Autodesk Inventor part; units mm, degrees
ref_plane "Work Plane2" through (2.8575, 0, 0) normal (1, 0, 0) x (0, 0, -1)
ref_plane "YZ Plane" through (0, 0, 0) normal (1, 0, 0) x (0, 1, 0)
ref_plane "XZ Plane" through (0, 0, 0) normal (0, 1, 0) x (-1, 0, 0)
ref_plane "Work Plane2" through (2.8575, 0, 0) normal (1, 0, 0) x (0, 0, -1)
sketch "Sketch6" plane through (2.8575, 0, 0) normal (1, 0, 0) x (0, 0, -1)
  line L0 (0.7654, -5.6784) -> (0.7654, -5.022)
  line L1 (-0.7638, -5.6784) -> (-0.7638, -5.0222)
  arc A0 (5.6006, 2.3498) -> (5.5837, 2.3418) centre (6.3532, 0.7382) ccw
  arc A1 (-0.7638, -5.0222) -> (0.7654, -5.022) centre (0, 0) ccw
  line L2 (0.0008, -7.62) -> (-0.2439, -7.62)
  line L3 (0.0008, -7.62) -> (0.2479, -7.62)
  arc A2 (0.2479, -7.62) -> (0.7654, -5.6784) centre (-2.309, -5.8988) ccw
  arc A3 (-0.7638, -5.6784) -> (-0.2439, -7.62) centre (2.2185, -5.9201) ccw
  arc A4 (3.5877, -3.5965) -> (3.5976, -3.5866) centre (0, 0) ccw
  line L4 (3.502, -4.5349) -> (3.1738, -3.9665)
  line L5 (2.1777, -5.2996) -> (1.8496, -4.7313)
  arc A5 (1.8496, -4.7313) -> (3.1738, -3.9665) centre (0, 0) ccw
  line L6 (3.8107, -6.5987) -> (3.5988, -6.721)
  line L7 (3.8107, -6.5987) -> (4.0247, -6.4752)
  arc A6 (4.0247, -6.4752) -> (3.502, -4.5349) centre (0.9498, -6.263) ccw
  arc A7 (2.1777, -5.2996) -> (3.5988, -6.721) centre (4.8813, -4.0177) ccw
  line L8 (5.3003, -2.1764) -> (4.7319, -1.8482)
  line L9 (4.5358, -3.5007) -> (3.9675, -3.1726)
  arc A8 (3.9675, -3.1726) -> (4.7319, -1.8482) centre (0, 0) ccw
  line L10 (6.5995, -3.8093) -> (6.4772, -4.0212)
  line L11 (6.5995, -3.8093) -> (6.7231, -3.5953)
  arc A9 (6.7231, -3.5953) -> (5.3003, -2.1764) centre (3.954, -4.949) ccw
  arc A10 (4.5358, -3.5007) -> (6.4772, -4.0212) centre (6.2362, -1.0388) ccw
  line L12 (5.6784, 0.7654) -> (5.022, 0.7654)
  line L13 (5.6784, -0.7638) -> (5.0222, -0.7638)
  arc A11 (5.0222, -0.7638) -> (5.022, 0.7654) centre (0, 0) ccw
  line L14 (7.62, 0.0008) -> (7.62, -0.2439)
  line L15 (7.62, 0.0008) -> (7.62, 0.2479)
  arc A12 (7.62, 0.2479) -> (5.6784, 0.7654) centre (5.8988, -2.309) ccw
  arc A13 (5.6784, -0.7638) -> (7.62, -0.2439) centre (5.9201, 2.2185) ccw
  line L16 (4.5349, 3.502) -> (3.9665, 3.1738)
  line L17 (5.2996, 2.1777) -> (4.7313, 1.8496)
  arc A14 (4.7313, 1.8496) -> (3.9665, 3.1738) centre (0, 0) ccw
  line L18 (6.5987, 3.8107) -> (6.721, 3.5988)
  line L19 (6.5987, 3.8107) -> (6.4752, 4.0247)
  arc A15 (6.4752, 4.0247) -> (4.5349, 3.502) centre (6.263, 0.9498) ccw
  arc A16 (5.2996, 2.1777) -> (6.721, 3.5988) centre (4.0177, 4.8813) ccw
  line L20 (2.1764, 5.3003) -> (1.8482, 4.7319)
  line L21 (3.5007, 4.5358) -> (3.1726, 3.9675)
  arc A17 (3.1726, 3.9675) -> (1.8482, 4.7319) centre (0, 0) ccw
  line L22 (3.8093, 6.5995) -> (4.0212, 6.4772)
  line L23 (3.8093, 6.5995) -> (3.5953, 6.7231)
  arc A18 (3.5953, 6.7231) -> (2.1764, 5.3003) centre (4.949, 3.954) ccw
  arc A19 (3.5007, 4.5358) -> (4.0212, 6.4772) centre (1.0388, 6.2362) ccw
  line L24 (-0.7654, 5.6784) -> (-0.7654, 5.022)
  line L25 (0.7638, 5.6784) -> (0.7638, 5.0222)
  arc A20 (0.7638, 5.0222) -> (-0.7654, 5.022) centre (0, 0) ccw
  line L26 (-0.0008, 7.62) -> (0.2439, 7.62)
  line L27 (-0.0008, 7.62) -> (-0.2479, 7.62)
  arc A21 (-0.2479, 7.62) -> (-0.7654, 5.6784) centre (2.309, 5.8988) ccw
  arc A22 (0.7638, 5.6784) -> (0.2439, 7.62) centre (-2.2185, 5.9201) ccw
  line L28 (-3.502, 4.5349) -> (-3.1738, 3.9665)
  line L29 (-2.1777, 5.2996) -> (-1.8496, 4.7313)
  arc A23 (-1.8496, 4.7313) -> (-3.1738, 3.9665) centre (0, 0) ccw
  line L30 (-3.8107, 6.5987) -> (-3.5988, 6.721)
  line L31 (-3.8107, 6.5987) -> (-4.0247, 6.4752)
  arc A24 (-4.0247, 6.4752) -> (-3.502, 4.5349) centre (-0.9498, 6.263) ccw
  arc A25 (-2.1777, 5.2996) -> (-3.5988, 6.721) centre (-4.8813, 4.0177) ccw
  line L32 (-5.3003, 2.1764) -> (-4.7319, 1.8482)
  line L33 (-4.5358, 3.5007) -> (-3.9675, 3.1726)
  arc A26 (-3.9675, 3.1726) -> (-4.7319, 1.8482) centre (0, 0) ccw
  line L34 (-6.5995, 3.8093) -> (-6.4772, 4.0212)
  line L35 (-6.5995, 3.8093) -> (-6.7231, 3.5953)
  arc A27 (-6.7231, 3.5953) -> (-5.3003, 2.1764) centre (-3.954, 4.949) ccw
  arc A28 (-4.5358, 3.5007) -> (-6.4772, 4.0212) centre (-6.2362, 1.0388) ccw
  line L36 (-5.6784, -0.7654) -> (-5.022, -0.7654)
  line L37 (-5.6784, 0.7638) -> (-5.0222, 0.7638)
  arc A29 (-5.0222, 0.7638) -> (-5.022, -0.7654) centre (0, 0) ccw
  line L38 (-7.62, -0.0008) -> (-7.62, 0.2439)
  line L39 (-7.62, -0.0008) -> (-7.62, -0.2479)
  arc A30 (-7.62, -0.2479) -> (-5.6784, -0.7654) centre (-5.8988, 2.309) ccw
  arc A31 (-5.6784, 0.7638) -> (-7.62, 0.2439) centre (-5.9201, -2.2185) ccw
  line L40 (-4.5349, -3.502) -> (-3.9665, -3.1738)
  line L41 (-5.2996, -2.1777) -> (-4.7313, -1.8496)
  arc A32 (-4.7313, -1.8496) -> (-3.9665, -3.1738) centre (0, 0) ccw
  line L42 (-6.5987, -3.8107) -> (-6.721, -3.5988)
  line L43 (-6.5987, -3.8107) -> (-6.4752, -4.0247)
  arc A33 (-6.4752, -4.0247) -> (-4.5349, -3.502) centre (-6.263, -0.9498) ccw
  arc A34 (-5.2996, -2.1777) -> (-6.721, -3.5988) centre (-4.0177, -4.8813) ccw
  line L44 (-2.1764, -5.3003) -> (-1.8482, -4.7319)
  line L45 (-3.5007, -4.5358) -> (-3.1726, -3.9675)
  arc A35 (-3.1726, -3.9675) -> (-1.8482, -4.7319) centre (0, 0) ccw
  line L46 (-3.8093, -6.5995) -> (-4.0212, -6.4772)
  line L47 (-3.8093, -6.5995) -> (-3.5953, -6.7231)
  arc A36 (-3.5953, -6.7231) -> (-2.1764, -5.3003) centre (-4.949, -3.954) ccw
  arc A37 (-3.5007, -4.5358) -> (-4.0212, -6.4772) centre (-1.0388, -6.2362) ccw
  arc A38 (-1.8482, -4.7319) -> (-0.7638, -5.0222) centre (0, 0) ccw
  line L48 (-2.0137, 5.0155) -> (-0.7654, 5.3502)
  line L49 (0.7638, 5.3503) -> (2.0123, 5.0161)
  line L50 (3.3367, 4.2516) -> (4.2507, 3.3379)
  line L51 (5.0155, 2.0137) -> (5.3502, 0.7654)
  line L52 (5.3503, -0.7638) -> (5.0161, -2.0123)
  line L53 (4.2516, -3.3367) -> (3.3379, -4.2507)
  line L54 (2.0137, -5.0155) -> (0.7654, -5.3502)
  line L55 (-0.7638, -5.3503) -> (-2.0123, -5.0161)
  line L56 (-3.3367, -4.2516) -> (-4.2507, -3.3379)
  line L57 (-5.0155, -2.0137) -> (-5.3502, -0.7654)
  line L58 (-5.3503, 0.7638) -> (-5.0161, 2.0123)
  line L59 (-4.2516, 3.3367) -> (-3.3379, 4.2507)
  circle A39 centre (0, 0) radius 5.0531
  point P0 (0, 0)
  point P1 (-4.2516, 3.3367)
  dimension "d94" = 360
extrude "Extrusion19" add sketch "Sketch6" against normal blind 5.7277 contours A2 L3 L2 A3 L1 A1 L0 | L0 A1 A38 A35 L45 L56 L40 A32 L41 L57 L36 A29 L37 L58 L32 A26 L33 L59 L28 A23 L29 L48 L24 A20 L25 L49 L20 A17 L21 L50 L16 A14 L17 L51 L12 A11 L13 L52 L8 A8 L9 L53 L4 A5 L5 L54 | L5 A5 L4 A6 L7 L6 A7 | L1 L55 L44 A38 | L44 A36 L47 L46 A37 L45 A35 | L9 A8 L8 A9 L11 L10 A10 | L40 A33 L43 L42 A34 L41 A32 | L13 A11 L12 A12 L15 L14 A13 | L36 A30 L39 L38 A31 L37 A29 | L17 A14 L16 A15 L19 L18 A16 | L32 A27 L35 L34 A28 L33 A26 | L21 A17 L20 A18 L23 L22 A19 | L28 A24 L31 L30 A25 L29 A23 | L25 A20 L24 A21 L27 L26 A22 | A39
sketch "Sketch7" plane through (-2.8702, 0, 0) normal (-1, 0, 0) x (0, 0, 1)
  circle A0 centre (0, 0) radius 2.286
  dimension "d104" = 4.572
extrude "Extrusion20" cut sketch "Sketch7" against normal blind 2540
sketch "Sketch8" plane through (-2.8702, 0, 0) normal (-1, 0, 0) x (0, 0, 1)
  circle A0 centre (0, 0) radius 5.08
  line L0 (-3.3367, 4.2516) -> (-4.2507, 3.3379)
  arc A1 (-4.2507, 3.3379) -> (-3.3367, 4.2516) centre (-4.209, 4.2103) ccw
  line L1 (-3.3367, 4.2516) -> (-3.5007, 4.5358)
  line L2 (-4.2507, 3.3379) -> (-3.3367, 4.2516)
  arc A2 (-5.3502, 0.7654) -> (-5.0155, 2.0137) centre (-5.7503, 1.5417) ccw
  line L3 (-5.3502, 0.7654) -> (-5.0155, 2.0137)
  arc A3 (-5.0161, -2.0123) -> (-5.3503, -0.7638) centre (-5.7507, -1.54) ccw
  line L4 (-5.0161, -2.0123) -> (-5.3503, -0.7638)
  arc A4 (-3.3379, -4.2507) -> (-4.2516, -3.3367) centre (-4.2103, -4.209) ccw
  line L5 (-3.3379, -4.2507) -> (-4.2516, -3.3367)
  arc A5 (-0.7654, -5.3502) -> (-2.0137, -5.0155) centre (-1.5417, -5.7503) ccw
  line L6 (-0.7654, -5.3502) -> (-2.0137, -5.0155)
  arc A6 (2.0123, -5.0161) -> (0.7638, -5.3503) centre (1.54, -5.7507) ccw
  line L7 (2.0123, -5.0161) -> (0.7638, -5.3503)
  arc A7 (4.2507, -3.3379) -> (3.3367, -4.2516) centre (4.209, -4.2103) ccw
  line L8 (4.2507, -3.3379) -> (3.3367, -4.2516)
  arc A8 (5.3502, -0.7654) -> (5.0155, -2.0137) centre (5.7503, -1.5417) ccw
  line L9 (5.3502, -0.7654) -> (5.0155, -2.0137)
  arc A9 (5.0161, 2.0123) -> (5.3503, 0.7638) centre (5.7507, 1.54) ccw
  line L10 (5.0161, 2.0123) -> (5.3503, 0.7638)
  arc A10 (3.3379, 4.2507) -> (4.2516, 3.3367) centre (4.2103, 4.209) ccw
  line L11 (3.3379, 4.2507) -> (4.2516, 3.3367)
  arc A11 (0.7654, 5.3502) -> (2.0137, 5.0155) centre (1.5417, 5.7503) ccw
  line L12 (0.7654, 5.3502) -> (2.0137, 5.0155)
  arc A12 (-2.0123, 5.0161) -> (-0.7638, 5.3503) centre (-1.54, 5.7507) ccw
  line L13 (-2.0123, 5.0161) -> (-0.7638, 5.3503)
  dimension "d107" = 10.16
  dimension "d110" = 360
extrude "Extrusion21" cut sketch "Sketch8" against normal blind 2540 contours A8 L9 | A7 L8 | A6 L7 | A5 L6 | A4 L5 | A3 L4 | A2 L3 | A1 L0 | A12 L13 | A11 L12 | A10 L11 | A9 L10
properties part number "Pinion final"
Work out the finished part from the listing and answer in its coordinate system (mm). A direction names the side the tool comes from. Give positions to 0.01 mm unless a question says otherwise; leave off trailing zeros. Loops run counter-clockwise (first coordinate to the right, second up) from the corner with the lowest first, then second, coordinate; pieces in that order, holes last. Notation, with made-up numbers: (54.5, 42.25) -> (68.5, 42.25) arc R29 cw to (68.5, 67.25) -> close; hole circle Ø10 at (11.25, -33.75). An arc over 180 degrees is marked (long way). One line per question, with ' | ' between items. Start each with the question number.
1) For faces 4 (the face through (0.034, -2.777, -6.141)), 5 (the face through (0.034, -3.925, -5.448)), 6 (the face through (-0.046, 3.585, -3.599)), determine the directions among +Z, -Z, +X, -X, +Y, -Y from which every point of the face is accessible in a straight line to the end or side of a thin tool.
2) Each of these flat-tipped pins is pushed along its axis until it touches: pin 1 (2 mm diameter, centred on x = 1.5, y = -4, fed in from +Z); pin 2 (1 mm diameter, centred on x = 0.5, y = -5.5, fed in from +Z); pin 3 (2 mm diameter, centred on x = -1.5, z = -4, fed in from -Y). Where does it stop, or does it pass through?
3) Straight lines are drawn through the part: L1, parallel to Y at x = -0.65, z = 0; L2, parallel to Z at x = -1.2, y = 5.5; L3, parallel to Z at x = -1.1, y = 5. For each, find the intervals that lie inside material, in ascending order.
4) Section A-A, the plane y = 0 is taken. Determine the outline of the cut face in (x, z), then the cut area to 3 significant figures.
5) Determine the mould class of faces 1 (the face through (0.034, -2.755, 6.123)), 2 (the face through (0.034, 2.755, -6.123)), 3 (the face through (-0.046, 3.599, 3.585)) for opening direction Z: +Z half, -Z half, draft (parallel to the pull), parting line (faces both ways), or undercut.
Resolved:
1) face 4: -Z, +X, -X | face 5: +X, -X, -Y | face 6: +X, -X
2) pin 1: z = 6.72 | pin 2: z = 4.02 | pin 3: y = -6.72
3) L1: -7.62 to -2.29, 2.29 to 7.62 | L2: -3.94 to -2.28, -0.76 to 0.77, 2.28 to 3.94 | L3: -3.76 to -1.99, -1.09 to 1.09, 1.99 to 3.76
4) outline: (-2.87, -7.62) -> (2.86, -7.62) -> (2.86, -2.29) -> (-2.87, -2.29) -> close; (-2.87, 2.29) -> (2.86, 2.29) -> (2.86, 7.62) -> (-2.87, 7.62) -> close | area: 61.1 mm2
5) face 1: +Z half | face 2: -Z half | face 3: undercut
